Can you work these out from the drawing? Everything is in mm from the part's minimum corner. Round coordinates to 2 decimals unless told otherwise and drop trailing zeros. Order: outer loops, then holes, each group sorted by start corner. A loop starts at its lowest first (then second) coordinate and runs counter-clockwise, first axis right, second up. Notation, with made-up numbers: (-13.75, -3.5) -> (44.25, -3.5) arc R16 cw to (44.25, 18.5) -> close; hole circle Ø11 at (-31.75, 71.25). An arc over 180 degrees is marked (long way). One line per item, written item: value.
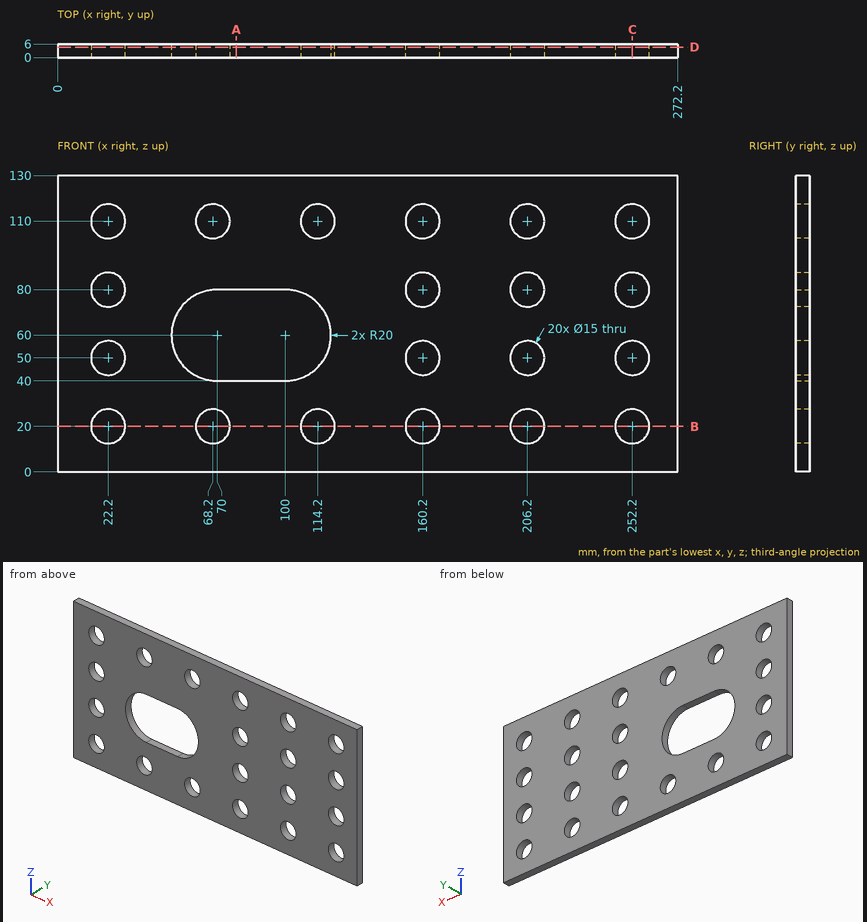
Q1. I want a section at A-A on x = 78.5. List the corners of the cut face in (y, z) for me.
Answers below:
outline: (0, 0) -> (6, 0) -> (6, 40) -> (0, 40) -> close; (0, 80) -> (6, 80) -> (6, 130) -> (0, 130) -> close
Q2. Please list where these lines run through material, in increasing order: line 1 along Z through (x, y) = (160.2, 3.15); line 2 along Z through (x, y) = (68.2, 3.1); line 3 along Z through (x, y) = (110, 4.3).
Answers below:
line 1: 0 to 12.5, 27.5 to 42.5, 57.5 to 72.5, 87.5 to 102.5, 117.5 to 130
line 2: 0 to 12.5, 27.5 to 40.08, 79.92 to 102.5, 117.5 to 130
line 3: 0 to 13.79, 26.21 to 42.68, 77.32 to 103.79, 116.21 to 130
Q3. Will these pins go through, and if not, where does the flat tip stop? pin 1 Ø17 at (x, z) = (160.2, 80) entering from +Y; pin 2 Ø12 at (x, z) = (160.2, 20) entering from -Y.
Answers below:
pin 1: y = 6
pin 2: through
Q4. I want a section at D-D on y = 4.65. Give the number of separate pieces and of enclosed holes in the cut face, plus the area to 3 significant figures.
Answers below:
separate pieces: 1
enclosed holes: 21
area: 29,400 mm^2
Q5. I want a section at C-C on x = 252.2. List the corners of the cut face in (y, z) for me, plus the area to 3 significant figures.
Answers below:
outline: (0, 0) -> (6, 0) -> (6, 12.5) -> (0, 12.5) -> close; (0, 27.5) -> (6, 27.5) -> (6, 42.5) -> (0, 42.5) -> close; (0, 57.5) -> (6, 57.5) -> (6, 72.5) -> (0, 72.5) -> close; (0, 87.5) -> (6, 87.5) -> (6, 102.5) -> (0, 102.5) -> close; (0, 117.5) -> (6, 117.5) -> (6, 130) -> (0, 130) -> close
area: 420 mm^2
Q6. I want a section at B-B on z = 20. List the corners of the cut face in (x, y) for me.
Answers below:
outline: (0, 0) -> (14.7, 0) -> (14.7, 6) -> (0, 6) -> close; (29.7, 0) -> (60.7, 0) -> (60.7, 6) -> (29.7, 6) -> close; (75.7, 0) -> (106.7, 0) -> (106.7, 6) -> (75.7, 6) -> close; (121.7, 0) -> (152.7, 0) -> (152.7, 6) -> (121.7, 6) -> close; (167.7, 0) -> (198.7, 0) -> (198.7, 6) -> (167.7, 6) -> close; (213.7, 0) -> (244.7, 0) -> (244.7, 6) -> (213.7, 6) -> close; (259.7, 0) -> (272.2, 0) -> (272.2, 6) -> (259.7, 6) -> close
